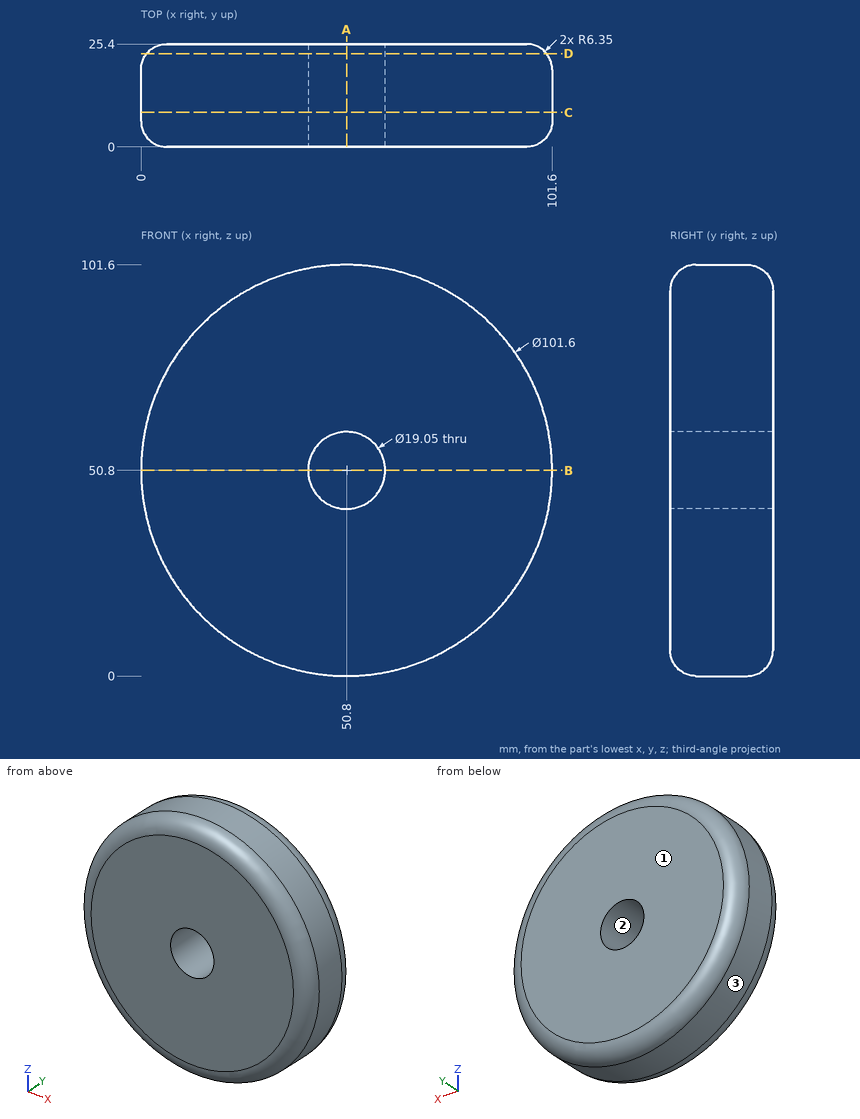
Check sheet for the drawn part. Datum: minimum x, y, z corner. Units: mm. Give positions to 0.01 mm unless a question says otherwise; leave off trailing zeros. Order: outer loops, then holes, each group sorted by start corner. A loop starts at its lowest first (then second) coordinate and runs counter-clockwise, first axis right, second up. Notation, with made-up numbers: (60, -12) - (76, -12) arc R23 cw to (76, 21) - close; hole circle Ø4 at (50.5, 27). An arc over 180 degrees is marked (long way). Write item = value, one per line. Start each with the question number.
1) Section check B-B (z = 50.8). Enter the section's corners in (x, y) (3 decimals), then the cut area to 3 significant figures.
2) Scan lines: L1, parallel to X at y = 9.5, z = 52; L2, parallel to X at y = 14.5, z = 15.5; L3, parallel to Z at x = 12, y = 21.5. Record each from-to range of solid material in increasing order.
3) Section check D-D (y = 23). Enter the section's corners in (x, z) (3 decimals), then the cut area to 3 significant figures.
4) Draft check along X on the marked faces 1, 2 and 3. Enter one of: released by +X, released by -X, zero draft, split by the parting line, or undercut.
5) Gauge pin test, flat ends, axial feed: pin 1 Ø2 at (y, z) = (14, 82.5) entering from -X; pin 2 Ø10 at (y, z) = (14.5, 16.5) entering from +X; pin 3 Ø2 at (x, y) = (20.5, 9.5) entering from -Z. Record the tip position at first contact, or that the pin passes through.
6) Section check C-C (y = 8.5). Enter the section's corners in (x, z) (3 decimals).
7) Section check A-A (x = 50.8). Enter the section's corners in (y, z) (3 decimals), then the cut area to 3 significant figures.
Geometry check:
q1.outline = (0, 6.35) arc R6.35 ccw to (6.35, 0) - (41.275, 0) - (41.275, 25.4) - (6.35, 25.4) arc R6.35 ccw to (0, 19.05) - close; (60.325, 0) - (95.25, 0) arc R6.35 ccw to (101.6, 6.35) - (101.6, 19.05) arc R6.35 ccw to (95.25, 25.4) - (60.325, 25.4) - close
q1.area = 2,060 mm2
q2.L1 = 0.01 to 41.35, 60.25 to 101.59
q2.L2 = 14.27 to 87.33
q2.L3 = 18.78 to 82.82
q3.outline = circle Ø98.844 at (50.8, 50.8); hole circle Ø19.05 at (50.8, 50.8)
q3.area = 7,390 mm2
q4.face_1 = zero draft
q4.face_2 = undercut
q4.face_3 = split by the parting line
q5.pin_1 = 10.33
q5.pin_2 = 92.3
q5.pin_3 = 9.3
q6.outline = circle Ø101.6 at (50.8, 50.8); hole circle Ø19.05 at (50.8, 50.8)
q7.outline = (0, 6.35) arc R6.35 ccw to (6.35, 0) - (19.05, 0) arc R6.35 ccw to (25.4, 6.35) - (25.4, 41.275) - (0, 41.275) - close; (0, 60.325) - (25.4, 60.325) - (25.4, 95.25) arc R6.35 ccw to (19.05, 101.6) - (6.35, 101.6) arc R6.35 ccw to (0, 95.25) - close
q7.area = 2,060 mm2
